Here's how the part is built. I have some questions about the finished solid (model axes, mm). Face numbers are marked on the shaded views. A direction names the side the tool comes from. Coordinates: 2 decimals unless noted, no trailing zeros. Write each loop counter-clockwise with the first axis right and the second up, starting at its lowest first coordinate (ties: lowest second). Pieces come first, ordered by that corner, then holes. Notation, with made-up numbers: (-33, 86) -> (19, 86) arc R27 cw to (19, 123) -> close; hole circle Ø5 at (81.25, 14.5). An arc over 180 degrees is marked (long way). Use a Markdown table: item, result. Add a question column.
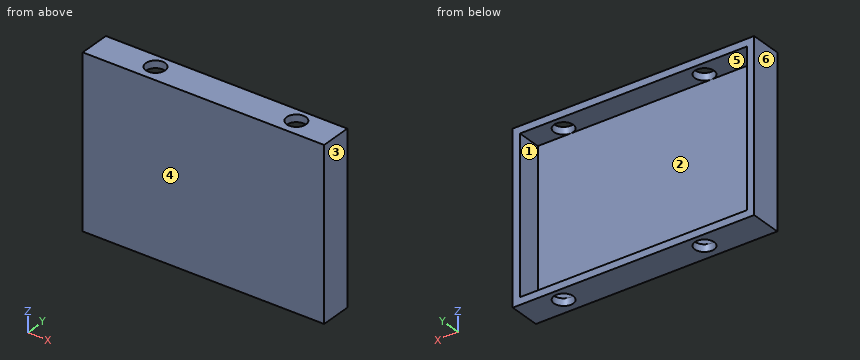
```python
from build123d import *

# Parameters (mm, degrees)
CROQUIS1_W              = 500
CROQUIS1_H              = 350
SALIENTE_EXTRUIR1_DEPTH = 15
CROQUIS2_W              = 500
CROQUIS2_H              = 350
CROQUIS2_W_2            = 470
CROQUIS2_H_2            = 320
SALIENTE_EXTRUIR2_DEPTH = 50
CROQUIS3_R              = 20
CORTAR_EXTRUIR1_DEPTH   = 351


with BuildPart() as part:
    # Croquis1 → Saliente-Extruir1 (new body)
    with BuildSketch(Plane(origin=(0, 0, 0), x_dir=(1, 0, 0), z_dir=(0, 1, 0))):
        Rectangle(CROQUIS1_W, CROQUIS1_H)
    extrude(amount=SALIENTE_EXTRUIR1_DEPTH)

    # Croquis2 → Saliente-Extruir2 (add)
    with BuildSketch(Plane(origin=(0, 15, 0), x_dir=(1, 0, 0), z_dir=(0, 1, 0))):
        Rectangle(CROQUIS2_W, CROQUIS2_H)
        Rectangle(CROQUIS2_W_2, CROQUIS2_H_2, mode=Mode.SUBTRACT)
    extrude(amount=SALIENTE_EXTRUIR2_DEPTH)

    # Croquis3 → Cortar-Extruir1 (cut, through all)
    with BuildSketch(Plane.XY.offset(175)):
        with Locations((-125, 35)):
            Circle(CROQUIS3_R)
        with Locations((166.666666667, 35)):
            Circle(CROQUIS3_R)
    extrude(amount=-CORTAR_EXTRUIR1_DEPTH, mode=Mode.SUBTRACT)


solid = part.part
```
Q1. Will these pins go through, and if not, where does the flat tip stop? pin 1 (12 mm diameter, centred on x = 18.5, z = -127, fed in from +Y); pin 2 (24 mm diameter, centred on x = 166.67, y = 35, fed in from -Z) (3 decimals); pin 3 (8 mm diameter, centred on x = 95.5, z = -91, fed in from -Y).
Q2. Suppose I cut it at B-B, the plane z = 29.5. Write out the boundary of the cut face in (x, y), and give its area (3 significant figures).
Q3. Which directions (+Z, -Z, +X, -X, +Y, -Y) give clear straight access to the entire face, cutting with the end or side of a thin tool? Please do the marked faces 5 and 6.
Q4. Suppose I cut it at C-C, the plane x = -152.5. Write out the boundary of the cut face in (y, z).
Q5. Thinking about a two-plate mould opening in X: for the marked faces 1, 2, 3 and 4, which applies, released by +X, released by -X, zero draft, split by the parting line, or undercut?
Q6. Please list where these lines run through material, in increasing order: line 1 (X direction, y = 35, z = -171); line 2 (X direction, y = 27, z = -54); line 3 (Z direction, x = 204.5, y = 24.5).
Q7. Suppose I cut it at A-A, the plane y = 35. Write out the boundary of the cut face in (x, z).
Answer key:
| question | item | result |
|---|---|---|
| 1 | pin 1 | stops at y = 15 |
| 1 | pin 2 | passes through |
| 1 | pin 3 | stops at y = 0 |
| 2 | outline | (-250, 0) -> (250, 0) -> (250, 65) -> (235, 65) -> (235, 15) -> (-235, 15) -> (-235, 65) -> (-250, 65) -> close |
| 2 | area | 9,000 mm^2 |
| 3 | face 5 | +Y |
| 3 | face 6 | +Z, -Z, -X, +Y, -Y |
| 4 | outline | (0, -175) -> (65, -175) -> (65, -160) -> (15, -160) -> (15, 160) -> (65, 160) -> (65, 175) -> (0, 175) -> close |
| 5 | face 1 | undercut |
| 5 | face 2 | undercut |
| 5 | face 3 | released by +X |
| 5 | face 4 | zero draft |
| 6 | line 1 | x = -250 to -145, -105 to 146.67, 186.67 to 250 |
| 6 | line 2 | x = -250 to -235, 235 to 250 |
| 6 | line 3 | z = -175 to -160, 160 to 175 |
| 7 | outline | (-250, -175) -> (-145, -175) -> (-145, -160) -> (-235, -160) -> (-235, 160) -> (-145, 160) -> (-145, 175) -> (-250, 175) -> close; (-105, -175) -> (146.67, -175) -> (146.67, -160) -> (-105, -160) -> close; (-105, 160) -> (146.67, 160) -> (146.67, 175) -> (-105, 175) -> close; (186.67, -175) -> (250, -175) -> (250, 175) -> (186.67, 175) -> (186.67, 160) -> (235, 160) -> (235, -160) -> (186.67, -160) -> close |
